Autodesk Inventor part; units mm, degrees
ref_plane "YZ Plane" through (0, 0, 0) normal (1, 0, 0) x (0, 1, 0)
ref_plane "XZ Plane" through (0, 0, 0) normal (0, 1, 0) x (-1, 0, 0)
ref_plane "XY Plane" through (0, 0, 0) normal (0, 0, 1) x (1, 0, 0)
sketch "Profile" plane through (0, 0, 0) normal (0, 0, 1) x (1, 0, 0)
  circle A0 centre (-41.4125, 89.9251) radius 3.175
  circle A1 centre (-27.9037, 3.7025) radius 1.5875
  circle A2 centre (-27.8803, -10.7935) radius 1.5875
  circle A3 centre (-13.3843, -10.7935) radius 1.5875
  circle A4 centre (72.5232, -75.6183) radius 3.175
  line L0 (-43.1149, 99.546) -> (-34.6506, 95.599)
  line L1 (-34.6506, 95.599) -> (-23.2362, 53)
  line L2 (-23.2362, 53) -> (79.5232, -33.2254)
  line L3 (-43.1149, 99.546) -> (-59.4044, 83.2171)
  line L4 (-59.4044, 83.2171) -> (-59.3372, 27.6567)
  line L5 (-59.3372, 27.6567) -> (-30.5183, -15.7204)
  line L6 (-30.5183, -15.7204) -> (17.4817, -15.6624)
  line L7 (65.5232, -82.6183) -> (79.5232, -82.6183)
  line L8 (79.5232, -82.6183) -> (79.5232, -33.2254)
  line L9 (17.4817, -15.6624) -> (52.5232, -45.0657)
  line L10 (-87.1899, 0) -> (107.3087, 0) construction
  line L11 (0, -119.0512) -> (0, 135.9789) construction
  line L12 (-36.2503, -15.7274) -> (-46.8807, -15.7402) construction
  line L13 (-41.4125, 89.9251) -> (-41.2847, -15.7335) construction
  line L14 (72.5232, -75.6183) -> (72.5232, 0) construction
  line L15 (72.5232, -75.6183) -> (0, -75.6183) construction
  line L16 (-41.4125, 89.9251) -> (0, 89.9251) construction
  line L17 (-23.2362, 53) -> (-59.3372, 27.6567) construction
  line L18 (23.9517, -13.8645) -> (32.6799, -3.0672)
  line L19 (-15.6986, 30.74) -> (-10.1602, 32.89)
  line L20 (-10.1602, 32.89) -> (27.3216, 1.4391)
  line L21 (-15.6986, 30.74) -> (-19.2013, 8.0713)
  line L22 (-19.2013, 8.0713) -> (-5.274, -8.6899)
  line L23 (-5.274, -8.6899) -> (19.1575, -8.6603)
  line L24 (19.1575, -8.6603) -> (27.3216, 1.4391)
  line L25 (-25.993, 13.7438) -> (-23.435, 30.2982)
  line L26 (-23.435, 30.2982) -> (-25.4448, 35.4753)
  line L27 (-25.4448, 35.4753) -> (-37.872, 45.903)
  line L28 (-49.7674, 30.8778) -> (-36.5022, 10.9116)
  line L29 (-36.5022, 10.9116) -> (-25.993, 13.7438)
  line L30 (-49.7674, 30.8778) -> (-49.7855, 45.8886)
  line L31 (-49.7855, 45.8886) -> (-37.872, 45.903)
  line L32 (52.5232, -45.0657) -> (52.5232, -71.7101)
  line L33 (52.5232, -71.7101) -> (65.5232, -82.6183)
  line L34 (-38.6692, 52.7662) -> (-33.1987, 57.5138)
  line L35 (-33.1987, 57.5138) -> (-38.5608, 77.5256)
  line L36 (-38.5608, 77.5256) -> (-47.0549, 81.4864)
  line L37 (-47.0549, 81.4864) -> (-51.5318, 77.2647)
  line L38 (-51.5318, 77.2647) -> (-51.5078, 57.4488)
  line L39 (-51.5078, 57.4488) -> (-46.8759, 52.7563)
  line L40 (-46.8759, 52.7563) -> (-38.6692, 52.7662)
  line L41 (32.6799, -3.0672) -> (45.3602, -13.8645)
  line L42 (45.3602, -13.8645) -> (23.9517, -13.8645)
  line L43 (32.6799, -21.3341) -> (52.5232, -21.3341)
  line L44 (32.6799, -21.3341) -> (52.5232, -35.6319)
  line L45 (52.5232, -35.6319) -> (52.5232, -21.3341)
  line L46 (58.4785, -46.424) -> (59.1425, -69.4967)
  line L47 (59.1425, -69.4967) -> (76.4098, -45.908)
  line L48 (76.4098, -45.908) -> (58.4785, -46.424)
  line L49 (57.3166, -38.9544) -> (58.6445, -24.0152)
  line L50 (58.6445, -24.0152) -> (73.2517, -36.7965)
  line L51 (73.2517, -36.7965) -> (57.3166, -38.9544)
  point P0 (0, 0)
  point P1 (65.5232, -75.6183)
  point P2 (-16, 37.7902)
  point P3 (-51.3919, 28.3472)
  point P4 (-34.7148, 3.2455)
  point P5 (-52.349, 37.4497)
  point P6 (-29.1922, 43.0466)
  dimension "d0" = 7
  dimension "d1" = 7
  dimension "d3" = 8
  dimension "d4" = 8
  dimension "d5" = 8
  dimension "d6" = 65
  dimension "d7" = 15
  dimension "d8" = 45
  dimension "d12" = 145
  dimension "d17" = 18
  dimension "d37" = 35
  dimension "d56" = 53
  dimension "d63" = 7
  dimension "d65" = 120
  dimension "d66" = 7
  dimension "d68" = 20
  dimension "d69" = 48
  dimension "d70" = 4.9237
extrude "Plate1" add sketch "Profile" along normal blind 3.048
fillet "OutsideFilletsFeature" radius 6 10 edges at (65.5232, -82.6183, 1.524) (79.5232, -82.6183, 1.524) (-43.1149, 99.546, 1.524) (-34.6506, 95.599, 1.524) (-59.4044, 83.2171, 1.524) (-23.2362, 53, 1.524) (-59.3372, 27.6567, 1.524) (-30.5183, -15.7204, 1.524) (17.4817, -15.6624, 1.524) (79.5232, -33.2254, 1.524)
equation "\"d1\" = d0"
equation "\"d4\" = d3"
equation "\"d5\" = d3"
equation "\"BendRadius\" = Thickness"
equation "\"BendReliefWidth\" = Thickness"
equation "\"BendReliefDepth\" = 0.5 * Thickness"
equation "\"CornerReliefSize\" = 4 * Thickness"
equation "\"MinimumRemnant\" = 2 * Thickness"
equation "\"TransitionRadius\" = BendRadius"
equation "\"JacobiRadiusSize\" = BendRadius"
equation "\"GapSize\" = Thickness"
properties part number "ShoulderBracketRedesign"
Can you work these out from the model? Positions are in its coordinate system, mm. A direction names the side the tool comes from. Give positions to 0.01 mm unless a question says otherwise; leave off trailing zeros. Order: outer loops, then holes, each group sorted by start corner. A loop starts at its lowest first (then second) coordinate and runs counter-clockwise, first axis right, second up. Notation, with made-up numbers: (12.5, 74.25) - (54.5, 74.25) arc R10 cw to (54.5, 79.25) - close; hole circle Ø4 at (19.5, 78). An arc over 180 degrees is marked (long way). Write each question's results on one line, items separated by ' | '.
1) If we mould it in two halves opening along Y, with no side actions, what happens to faces 3 (the face through (77.719, -80.907, 1.545)), 4 (the face through (-51.79, 90.85, 1.5)), 5 (the face through (-42.101, 93.025, 1.503))? For each: pulls with the +Y half, pulls with the -Y half, needs draft (parallel to the pull), parting line crosses it, or undercut.
Final values:
face 3: pulls with the -Y half | face 4: pulls with the +Y half | face 5: undercut
2) On a 3-axis mill with a long thin cutter (end or side, diameter ignored), from which of +Z, -Z, +X, -X, +Y, -Y can I reach the whole of each face in a straight line? I mean faces 1 (the face through (8.3, 17.4, 1.5)), 2 (the face through (58.11, -76.4, 1.5)). Say none if no direction works.
Final values:
face 1: +Z, -Z | face 2: +Z, -Z, -X, -Y
3) Suppose I cut it at C-C, the plane z = 0.9. Give the number of separate pieces and of enclosed holes in the cut face, then the cut area to 3 significant figures.
Final values:
separate pieces: 1 | enclosed holes: 12 | area: 5,110 mm^2
4) Suppose I cut it at A-A, the plane y = -54.5. Write out the boundary of the cut face in (x, z).
Final values:
outline: (52.52, 0) - (58.71, 0) - (58.71, 3.05) - (52.52, 3.05) - close; (70.12, 0) - (79.52, 0) - (79.52, 3.05) - (70.12, 3.05) - close
5) I'm going to push flat-ended pins straight in: pin 1 Ø1.5 at (x, z) = (55, 0.5) entering from -Y; pin 2 Ø5 at (x, y) = (-13.38, -10.79) entering from +Z; pin 3 Ø1.5 at (x, z) = (35.5, 1.5) entering from +Y; pin 4 Ø0.9 at (y, z) = (-27.5, 1) entering from -X. Where does each tip first touch, or does it pass through?
Final values:
pin 1: stops at y = -74.42 | pin 2: stops at z = 3.05 | pin 3: stops at y = 4.34 | pin 4: stops at x = 31.05
6) Suppose I cut it at B-B, the plane x = 6.5. Write out the boundary of the cut face in (y, z), then the cut area to 3 significant figures.
Final values:
outline: (-15.68, 0) - (-8.68, 0) - (-8.68, 3.05) - (-15.68, 3.05) - close; (18.91, 0) - (28.05, 0) - (28.05, 3.05) - (18.91, 3.05) - close | area: 49.2 mm^2
7) Please list where these lines run through material, in increasing order: line 1 along Y through (x, z) = (37, 2.5); line 2 along Y through (x, z) = (25.5, 0.45); line 3 along X through (y, z) = (-34, 2.85). Write a range as [from, to].
Final values:
line 1: y = [-32.04, -24.45], [-21.33, -13.86], [-6.75, 2.46] | line 2: y = [-22.39, -13.86], [-11.95, -0.81], [2.97, 12.11] | line 3: x = [39.34, 50.26], [52.52, 57.76], [70.06, 79.17]
